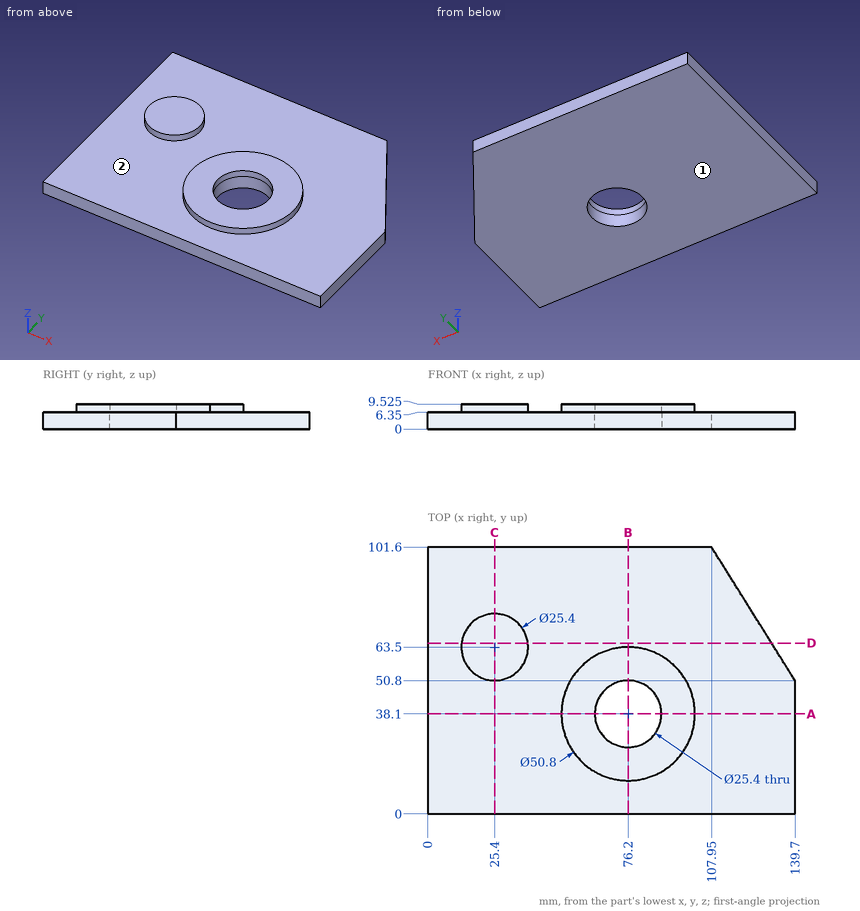
Part print with two shaded views. Sizes in mm from the minimum x, y, z corner. A direction names the side the tool comes from. Round coordinates to 2 decimals unless told otherwise and drop trailing zeros. Order: outer loops, then holes, each group sorted by start corner. A loop starts at its lowest first (then second) coordinate and runs counter-clockwise, first axis right, second up. Notation, with made-up numbers: (23.5, 82.25) - (69.5, 82.25) arc R33 cw to (69.5, 113.25) - close; hole circle Ø1 at (2.25, 46). An arc over 180 degrees is marked (long way). Answer in a Markdown table with one row per item. Add a question column.
(1) Drop a flat-ended pin along its axis: pin 1 Ø10 at (x, y) = (115.5, 34) entering from -Z. Give the stop position or say it passes through.
(2) 3-axis set-ups, long thin cutter, end or side, ignore diameter. For the marked faces 1 and 2: which of +Z, -Z, +X, -X, +Y, -Y reach the whole face in a straight line?
(3) Band-saw the part on D-D on y = 65. List the corners of the cut face in (x, z) (3 decimals), and give its area (3 significant figures).
(4) Probe L1, parallel to Y at x = 76.2, z = 8.75; L2, parallel to Y at x = 76.2, z = 3.25; L3, parallel to Z at x = 100.5, y = 27. List the from-to ranges inside material, lowest first. Write a range as [from, to].
(5) Band-saw the part on B-B on x = 76.2. List the corners of the cut face in (y, z) (3 decimals).
(6) Band-saw the part on C-C on x = 25.4. List the corners of the cut face in (y, z) (3 decimals).
(7) Band-saw the part on A-A on y = 38.1. List the corners of the cut face in (x, z) (3 decimals).
Data:
| question | item | result |
|---|---|---|
| 1 | pin 1 | stops at z = 0 |
| 2 | face 1 | -Z, +X, -X, +Y, -Y |
| 2 | face 2 | +Z |
| 3 | outline | (0, 0) - (130.825, 0) - (130.825, 6.35) - (38.011, 6.35) - (38.011, 9.525) - (12.789, 9.525) - (12.789, 6.35) - (0, 6.35) - close |
| 3 | area | 911 mm^2 |
| 4 | L1 | y = [12.7, 25.4], [50.8, 63.5] |
| 4 | L2 | y = [0, 25.4], [50.8, 101.6] |
| 4 | L3 | z = [0, 6.35] |
| 5 | outline | (0, 0) - (25.4, 0) - (25.4, 9.525) - (12.7, 9.525) - (12.7, 6.35) - (0, 6.35) - close; (50.8, 0) - (101.6, 0) - (101.6, 6.35) - (63.5, 6.35) - (63.5, 9.525) - (50.8, 9.525) - close |
| 6 | outline | (0, 0) - (101.6, 0) - (101.6, 6.35) - (76.2, 6.35) - (76.2, 9.525) - (50.8, 9.525) - (50.8, 6.35) - (0, 6.35) - close |
| 7 | outline | (0, 0) - (63.5, 0) - (63.5, 9.525) - (50.8, 9.525) - (50.8, 6.35) - (0, 6.35) - close; (88.9, 0) - (139.7, 0) - (139.7, 6.35) - (101.6, 6.35) - (101.6, 9.525) - (88.9, 9.525) - close |
